```python
from build123d import *

# Parameters (mm, degrees)
F1_DEPTH = 65.5
F2_W     = 26.5
F2_H     = 45.5
F3_DEPTH = 5
F4_R     = 6
F5_R     = 3


with BuildPart() as f1:
    # F0 (on Top) → F1 (new body)
    with BuildSketch(Plane.XY):
        Polygon((0, 2), (0, 0), (40, 0), (40, 20), (7.473088, 52.526912), (6.058875, 51.112698), (38, 19.171573), (38, 2), align=None)
    extrude(amount=F1_DEPTH)

    # F2 (on face) → F3 (cut)
    with BuildSketch(Plane(origin=(30, 30, 0), x_dir=(-0.707107, 0.707107, 0), z_dir=(0.707107, 0.707107, 0))):
        with Locations((9.107864, 32.75)):
            Rectangle(F2_W, F2_H)
    extrude(amount=-F3_DEPTH, mode=Mode.SUBTRACT)

    # F4
    f4_edges = [f1.edges().sort_by_distance(p)[0] for p in [
        (6.765981, 51.819805, 65.5),
        (6.765981, 51.819805, 0),
        (0, 1, 0),
        (0, 1, 65.5),
    ]]
    fillet(f4_edges, radius=F4_R)

    # F5
    f5_edges = [f1.edges().sort_by_distance(p)[0] for p in [
        (40, 20, 32.75),
        (38, 19.171573, 32.75),
        (38, 2, 32.75),
        (40, 0, 32.75),
    ]]
    fillet(f5_edges, radius=F5_R)


solid = f1.part
```
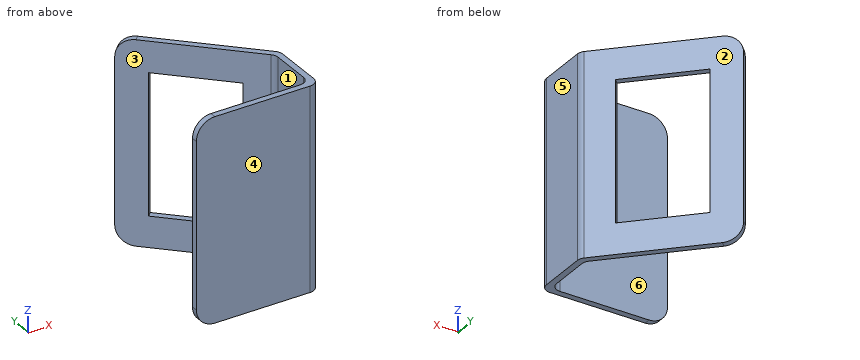
Check sheet for the modelled part. Datum: model origin and axes. Units: mm. Face numbers are marked on the shaded views. A direction names the side the tool comes from. Round coordinates to 2 decimals unless told otherwise and drop trailing zeros. Loops run counter-clockwise (first coordinate to the right, second up) from the corner with the lowest first, then second, coordinate; pieces in that order, holes last. Notation, with made-up numbers: (46, 17.25) - (53, 17.25) arc R16 ccw to (53, 25.25) - close; hole circle Ø3 at (26, 35.25). An arc over 180 degrees is marked (long way). Answer as a JSON object with one key per item and string values. Group by question number.
Q1. Sectioned sample at A-A, the plane z = 22. Enter the section's corners in (x, y), plus the area to 3 significant figures.
Q2. Sectioned sample at C-C, the plane y = 43.5. Enter the section's corners in (x, z).
Q3. Gauge pin test, flat ends, axial feed: P1, Ø1, axis at x = 4, z = 36.5, coming from the +Y side; P2, Ø8, axis at y = 8.5, z = 56.5, coming from the -X side. Record the tip position at first contact, or that the pin passes through.
Q4. Set-up check for the marked faces 5 and 6: record each of +Z, -Z, +X, -X, +Y, -Y from which the full face is reachable in a straight line by a thin tool's end or side.
Q5. Mould release check, pull along Y, two halves, no side actions. Record for the marked faces 1, 2, 3 and 4: released by +Y, released by -Y, zero draft, split by the parting line, or undercut.
Q6. Scan lines: line 1 along Y through (x, z) = (16, 46); line 2 along X through (y, z) = (18, 27.5); line 3 along Y through (x, z) = (32.5, 16). Record each from-to range of solid material in increasing order. Write a range as [from, to].
Q7. Sectioned sample at D-D, the plane y = 8. Enter the section's corners in (x, z).
Q8. Sectioned sample at B-B, the plane x = 22. Enter the section's corners in (y, z).
Solution:
{
 "1": {"outline": "(0, 0) - (37, 0) arc R3 ccw to (40, 3) - (40, 18.76) arc R3 ccw to (39.12, 20.88) - (32.93, 27.07) - (31.51, 25.66) - (37.12, 20.05) arc R3 cw to (38, 17.93) - (38, 5) arc R3 cw to (35, 2) - (0, 2) - close; (6.06, 51.11) - (12.78, 44.4) - (14.19, 45.81) - (7.47, 52.53) - close", "area": "153 mm²"},
 "2": {"outline": "(13.67, 0) - (16.5, 0) - (16.5, 10) - (13.67, 10) - close; (13.67, 55.5) - (16.5, 55.5) - (16.5, 65.5) - (13.67, 65.5) - close"},
 "3": {"P1": "stops at y = 2", "P2": "stops at x = 37.96"},
 "4": {"face 5": "+Z, -Z, +X, +Y, -Y", "face 6": "+Z, -Z, -X"},
 "5": {"face 1": "undercut", "face 2": "released by +Y", "face 3": "undercut", "face 4": "released by -Y"},
 "6": {"line 1": "y = [0, 2]", "line 2": "x = [38, 40]", "line 3": "y = [0, 2], [24.67, 26.64]"},
 "7": {"outline": "(38, 0) - (40, 0) - (40, 65.5) - (38, 65.5) - close"},
 "8": {"outline": "(0, 0) - (2, 0) - (2, 65.5) - (0, 65.5) - close; (35.17, 0) - (38, 0) - (38, 10) - (35.17, 10) - close; (35.17, 55.5) - (38, 55.5) - (38, 65.5) - (35.17, 65.5) - close"}
}
